from build123d import *

# Parameters (mm, degrees)
SKETCH_1_W          = 15
SKETCH_1_H          = 15
SKETCH_1_W_2        = 13
SKETCH_1_H_2        = 13
EXTRUDE_1_DEPTH     = 306.44
SKETCH_2_R          = 1.45
CUT_EXTRUDE_1_DEPTH = 307.898555878
SKETCH_3_R          = 1.45
CUT_EXTRUDE_2_DEPTH = 307.898555878


with BuildPart() as part:
    # 草图1 → 凸台-拉伸1 (new body)
    with BuildSketch(Plane(origin=(0, 0, 0), x_dir=(0, 0, -1), z_dir=(1, 0, 0))):
        Rectangle(SKETCH_1_W, SKETCH_1_H)
        Rectangle(SKETCH_1_W_2, SKETCH_1_H_2, mode=Mode.SUBTRACT)
    extrude(amount=EXTRUDE_1_DEPTH)

    # 草图2 → 切除-拉伸1 (cut, through all)
    with BuildSketch(Plane.XZ.offset(7.5)):
        with Locations(Location((110.44, 0, 0), (0, 0, 270))):
            Circle(SKETCH_2_R)
        with Locations(Location((210.44, 0, 0), (0, 0, 270))):
            Circle(SKETCH_2_R)
        with Locations(Location((283.44, 0, 0), (0, 0, 270))):
            Circle(SKETCH_2_R)
        with Locations(Location((296.94, 0, 0), (0, 0, 270))):
            Circle(SKETCH_2_R)
        with Locations(Location((150, 0, 0), (0, 0, 270))):
            Circle(SKETCH_2_R)
        with Locations(Location((160, 0, 0), (0, 0, 270))):
            Circle(SKETCH_2_R)
    extrude(amount=-CUT_EXTRUDE_1_DEPTH, mode=Mode.SUBTRACT)

    # 草图3 → 切除-拉伸2 (cut, through all)
    with BuildSketch(Plane(origin=(0, 0, -7.5), x_dir=(-1, 0, 0), z_dir=(0, 0, -1))):
        with Locations((-5, 0)):
            Circle(SKETCH_3_R)
        with Locations((-15, 0)):
            Circle(SKETCH_3_R)
    extrude(amount=-CUT_EXTRUDE_2_DEPTH, mode=Mode.SUBTRACT)


solid = part.part
Geometry check sheet. Reference: the model listing, model coordinates, mm. A direction names the side the tool comes from. Give positions to 0.01 mm unless a question says otherwise; leave off trailing zeros. Order: outer loops, then holes, each group sorted by start corner. A loop starts at its lowest first (then second) coordinate and runs counter-clockwise, first axis right, second up. Notation, with made-up numbers: (24, 77) - (52, 77) arc R18 cw to (52, 88) - close; hole circle Ø8 at (22, 45.5). An arc over 180 degrees is marked (long way). Answer as a JSON object with one key per item and string values.
(1) Cross-section at A-A (x = 65.5). Record the cut outline in (y, z), then the cut area to 3 significant figures.
Report:
{"outline": "(-7.5, -7.5) - (7.5, -7.5) - (7.5, 7.5) - (-7.5, 7.5) - close; hole (-6.5, -6.5) - (6.5, -6.5) - (6.5, 6.5) - (-6.5, 6.5) - close", "area": "56.0 mm^2"}
(2) Cross-section at B-B (y = -4). Record the cut outline in (x, z).
Report:
{"outline": "(0, -7.5) - (306.44, -7.5) - (306.44, -6.5) - (0, -6.5) - close; (0, 6.5) - (306.44, 6.5) - (306.44, 7.5) - (0, 7.5) - close"}
(3) Tool access check on faces 1 (the flat face through (151, 0, 6.5)), 2 (the flat face through (0, 0, 7)). Record the directions out of +Z, -Z, +X, -X, +Y, -Y that give a thin tool (end or side, any length) a straight path to the whole face; none if there is none.
Report:
{"face 1": "+X, -X", "face 2": "+Z, -Z, -X, +Y, -Y"}
(4) Material ranges on line 1 (Y direction, x = 103, z = -1.75); line 2 (Y direction, x = 5, z = 7.1), recorded low to high.
Report:
{"line 1": "-7.5 to -6.5, 6.5 to 7.5", "line 2": "-7.5 to -1.45, 1.45 to 7.5"}
(5) Depth check by flat-ended pin: pin 1 Ø1.7 at (x, z) = (296.94, 0) entering from +Y. Enter the tip coordinate at first touch or a pass-through.
Report:
{"pin 1": "through"}
(6) Draft check along Z on faces 3 (the flat face through (151, -7.5, 2)), 4 (the flat face through (151, 6.5, 2)), 5 (the flat face through (151, 0, -7.5)), 6 (the flat face through (151, 0, -6.5)). Enter one of: released by +Z, released by -Z, zero draft, split by the parting line, or undercut.
Report:
{"face 3": "zero draft", "face 4": "undercut", "face 5": "released by -Z", "face 6": "undercut"}
